Could you check a few things on this model? Use its own coordinates, in mm. A direction names the side the tool comes from. Give positions to 0.01 mm unless a question says otherwise; leave off trailing zeros. Loops run counter-clockwise (first coordinate to the right, second up) from the corner with the lowest first, then second, coordinate; pieces in that order, holes last. Notation, with made-up numbers: (62.25, 17) - (71.25, 17) arc R23 cw to (71.25, 32) - close; hole circle Ø3 at (-12, 48.25). An arc over 180 degrees is marked (long way). One line per item, written item: value. Start each with the question number.
Q1. I want a section at C-C (z = 3.25). Please give me the cut outline in (x, y), then the cut area to 3 significant figures.
Q2. I want a section at B-B (z = 1). Please give me the cut outline in (x, y), then the cut area to 3 significant figures.
Q3. I want a section at A-A (y = 6). Please give me the cut outline in (x, z).
Q4. I'm going to push flat-ended pins straight in: P1, Ø3, axis at y = 1.5, z = -2, coming from the +X side; P2, Ø1.5, axis at x = 9, y = 6.5, coming from the -Z side; P3, Ø5, axis at x = 13.5, y = 7, coming from the +Z side. Where does each tip first touch, or does it pass through?
Q5. For faces 1 (the face through (11.373, 7.464, -0.112)), 2 (the face through (-4, 12, 0)), which set-ups out of +Z, -Z, +X, -X, +Y, -Y let a thin tool reach every point of the face, with its end or its side?
Q6. If I drill on line 1 (X direction, y = 11, z = -4); line 2 (Z direction, x = 14.5, y = 5); line 3 (Y direction, x = 10, z = 1.5), over which ranges is the centre line in solid material (lowest first)? Write a range as from..to.
Q7. I want a section at D-D (y = 1.75). Please give me the cut outline in (x, z), then the cut area to 3 significant figures.
```python
from build123d import *

# Parameters (mm, degrees)
SKETCH1_W           = 21
SKETCH1_H           = 12
BOSS_EXTRUDE1_DEPTH = 12
BOSS_EXTRUDE2_DEPTH = 10


with BuildPart() as part:
    # Sketch1 → Boss-Extrude1 (new body)
    with BuildSketch(Plane(origin=(0, 0, 0), x_dir=(1, 0, 0), z_dir=(0, 1, 0))):
        with Locations((-4.056818182, -0.213068182)):
            Rectangle(SKETCH1_W, SKETCH1_H)
    extrude(amount=BOSS_EXTRUDE1_DEPTH)

    # Sketch2 → Boss-Extrude2 (add)
    with BuildSketch(Plane(origin=(6.443181818, 0, 0), x_dir=(0, 0, -1), z_dir=(1, 0, 0))):
        with BuildLine():
            ThreePointArc((1.286931818, 6), (-0.213068182, 7.5), (-1.713068182, 6))
            Line((-1.713068182, 6), (1.286931818, 6))
        make_face()
        with BuildLine():
            Line((1.286931818, 6), (-1.713068182, 6))
            ThreePointArc((-1.713068182, 6), (-0.213068182, 4.5), (1.286931818, 6))
        make_face()
    extrude(amount=BOSS_EXTRUDE2_DEPTH)


solid = part.part
```
Worked answers:
1. outline: (-14.56, 0) - (6.44, 0) - (6.44, 12) - (-14.56, 12) - close
1. area: 252 mm²
2. outline: (-14.56, 0) - (6.44, 0) - (6.44, 4.72) - (16.44, 4.72) - (16.44, 7.28) - (6.44, 7.28) - (6.44, 12) - (-14.56, 12) - close
2. area: 278 mm²
3. outline: (-14.56, -5.79) - (6.44, -5.79) - (6.44, -1.29) - (16.44, -1.29) - (16.44, 1.71) - (6.44, 1.71) - (6.44, 6.21) - (-14.56, 6.21) - close
4. P1: stops at x = 6.44
4. P2: stops at z = -1.29
4. P3: stops at z = 1.71
5. face 1: +X
5. face 2: +Z, -Z, +X, -X, +Y
6. line 1: x = -14.56..6.44
6. line 2: z = -0.9..1.33
6. line 3: y = 5.23..6.77
7. outline: (-14.56, -5.79) - (6.44, -5.79) - (6.44, 6.21) - (-14.56, 6.21) - close
7. area: 252 mm²
